Geometry: final body of the model. Coordinates: model frame, mm. A direction names the side the tool comes from. Give positions to 0.01 mm unless a question says otherwise; leave off trailing zeros. Write each loop counter-clockwise with the first axis right and the second up, starting at its lowest first coordinate (ties: lowest second). Pieces come first, ordered by that corner, then holes. Notation, with made-up numbers: M 19.25,-6 L 28.25,-6 A15 ccw 28.25,7 Z; hole C 14.5,55.25 d3. An arc over 180 degrees is marked long. Use one line per item in the form item = value. Start each with the question number.
Item 1: Section query C-C on z = -17. Return loops of the section in (x, y).
Item 2: Section query D-D on z = 0. Return loops of the section in (x, y).
Item 3: Section query A-A on x = -7. Return loops of the section in (y, z), then the cut area to 3 significant figures.
Item 4: Section query B-B on y = 4.25. Return loops of the section in (x, z).
Item 5: Access query for faces 4 (the flat face through (5, 0, 0)), 5 (the cylindrical face through (-4, -2, 0)), 6 (the flat face through (5, -0.5, -17.5)). Directions: +Z, -Z, +X, -X, +Y, -Y. A direction counts if a zero-diameter tool reaches every point of the face in a straight line with its end or side. Return the directions, or none.
Item 6: Pull-direction query (Y, two-part tool) for faces 1 (the flat face through (7, 0.1, 19)), 2 (the flat face through (-2, 0, 0)), 3 (the flat face through (0, 1, -5)); classes: released by +Y, released by -Y, zero draft, split by the parting line, or undercut.
Item 7: Contact query for flat-ended pins moving along their axis: P1, Ø1.5, axis at x = 3, z = 10.5, coming from the -Y side; P2, Ø4, axis at x = 8, z = -17.5, coming from the -Y side; P3, Ø1, axis at y = 4.5, z = -3.5, coming from the +X side. Output: stop coordinate, or through.
Item 8: Material intervals for line 1 along Z through (x, y) = (-2.75, 3); line 2 along X through (y, z) = (1.8, -17); line 3 along Z through (x, y) = (-3, 0), sorted ascending. Write a range as from..to.
from build123d import *

# Parameters (mm, degrees)
SKETCH_1_R          = 2
EXTRUDE_1_DEPTH     = 5
SKETCH_3_W          = 40
SKETCH_3_H          = 1.796813629
EXTRUDE_2_DEPTH     = 10
SKETCH_4_R          = 1.4
CUT_EXTRUDE_2_DEPTH = 20
SKETCH_6_R          = 2.5
EXTRUDE_3_DEPTH     = 7
SKETCH_7_R          = 2.8
SKETCH_7_R_2        = 2.2
CUT_EXTRUDE_3_DEPTH = 5
FILLET_1_R          = 1
EXTRUDE_START       = 5
SKETCH_8_W          = 5
SKETCH_8_H          = 4.9
SKETCH_8_R          = 1.4
EXTRUDE_4_DEPTH     = 5


with BuildPart() as part:
    # 스케치1 → 보스-돌출1 (new, symmetric)
    with BuildSketch(Plane(origin=(0, 0, 0), x_dir=(0, 0, -1), z_dir=(1, 0, 0))):
        Polygon((20, 6.896813629), (-20, 6.896813629), (-20, -1.103186371), (-15.1, -1.103186371), (-15.1, 5.1), (-5, 5.1), (-5, -3), (5, -3), (5, 5.1), (15.1, 5.1), (15.1, -1.103186371), (20, -1.103186371), align=None)
        Circle(SKETCH_1_R, mode=Mode.SUBTRACT)
    extrude(amount=EXTRUDE_1_DEPTH, both=True)

    # 스케치3 → 보스-돌출2 (add, symmetric)
    with BuildSketch(Plane(origin=(0, 0, 0), x_dir=(0, 0, -1), z_dir=(1, 0, 0))):
        with Locations((0, 5.998406815)):
            Rectangle(SKETCH_3_W, SKETCH_3_H)
    extrude(amount=EXTRUDE_2_DEPTH, both=True)

    # 스케치4 → 컷-돌출2 (cut)
    with BuildSketch(Plane(origin=(0, 0, 0), x_dir=(1, 0, 0), z_dir=(0, 1, 0))):
        with Locations(Location((-7, -17, 0), (0, 0, 90))):
            Circle(SKETCH_4_R)
        with Locations(Location((7, -17, 0), (0, 0, 90))):
            Circle(SKETCH_4_R)
        with Locations(Location((7, 17, 0), (0, 0, 90))):
            Circle(SKETCH_4_R)
        with Locations(Location((-7, 17, 0), (0, 0, 90))):
            Circle(SKETCH_4_R)
    extrude(amount=CUT_EXTRUDE_2_DEPTH, mode=Mode.SUBTRACT)

    # 스케치6 → 보스-돌출3 (add)
    with BuildSketch(Plane(origin=(5, 0, 0), x_dir=(0, 0, -1), z_dir=(1, 0, 0))):
        Circle(SKETCH_6_R)
    extrude(amount=-EXTRUDE_3_DEPTH)

    # 스케치7 → 컷-돌출3 (cut)
    with BuildSketch(Plane(origin=(5, 0, 0), x_dir=(0, 0, -1), z_dir=(1, 0, 0))):
        Circle(SKETCH_7_R)
        Circle(SKETCH_7_R_2, mode=Mode.SUBTRACT)
    extrude(amount=-CUT_EXTRUDE_3_DEPTH, mode=Mode.SUBTRACT)

    # 필렛1
    fillet_1_edges = [part.edges().sort_by_distance(p)[0] for p in [
        (5, 0, 2.2),
    ]]
    fillet(fillet_1_edges, radius=FILLET_1_R)

    # 스케치8 → 보스-돌출4 (add)
    # profile 1 of 4: a face of its own
    with BuildSketch(Plane.XZ.offset(-5.1).offset(EXTRUDE_START)):
        with Locations((-7.5, 17.55)):
            Rectangle(SKETCH_8_W, SKETCH_8_H)
        with Locations(Location((-7, 17, 0), (0, 0, 270))):
            Circle(SKETCH_8_R, mode=Mode.SUBTRACT)
    # profile 2 of 4: a face of its own
    with BuildSketch(Plane.XZ.offset(-5.1).offset(EXTRUDE_START)):
        with Locations((7.5, 17.55)):
            Rectangle(SKETCH_8_W, SKETCH_8_H)
        with Locations(Location((7, 17, 0), (0, 0, 270))):
            Circle(SKETCH_8_R, mode=Mode.SUBTRACT)
    # profile 3 of 4: a face of its own
    with BuildSketch(Plane.XZ.offset(-5.1).offset(EXTRUDE_START)):
        with Locations((-7.5, -17.55)):
            Rectangle(SKETCH_8_W, SKETCH_8_H)
        with Locations(Location((-7, -17, 0), (0, 0, 270))):
            Circle(SKETCH_8_R, mode=Mode.SUBTRACT)
    # profile 4 of 4: a face of its own
    with BuildSketch(Plane.XZ.offset(-5.1).offset(EXTRUDE_START)):
        with Locations((7.5, -17.55)):
            Rectangle(SKETCH_8_W, SKETCH_8_H)
        with Locations(Location((7, -17, 0), (0, 0, 270))):
            Circle(SKETCH_8_R, mode=Mode.SUBTRACT)
    extrude(amount=-EXTRUDE_4_DEPTH)


solid = part.part
Answer sheet:
q1.outline = M -10,0.1 L -8.4,0.1 L -8.4,6.9 L -10,6.9 Z; M -5.6,0.1 L -5,0.1 L -5,-1.1 L 5,-1.1 L 5,0.1 L 5.6,0.1 L 5.6,6.9 L -5.6,6.9 Z; M 8.4,0.1 L 10,0.1 L 10,6.9 L 8.4,6.9 Z
q2.outline = M -10,5.1 L -5,5.1 L -5,2 L -2,2 L -2,-2 L -5,-2 L -5,-3 L 5,-3 L 5,-2.8 L 0,-2.8 L 0,-2.2 L 4,-2.2 A1 ccw 5,-1.2 L 5,1.2 A1 ccw 4,2.2 L 0,2.2 L 0,2.8 L 5,2.8 L 5,5.1 L 10,5.1 L 10,6.9 L -10,6.9 Z
q3.outline = M 0.1,-20 L 6.9,-20 L 6.9,-18.4 L 0.1,-18.4 Z; M 0.1,-15.6 L 6.9,-15.6 L 6.9,15.6 L 0.1,15.6 L 0.1,15.1 L 5.1,15.1 L 5.1,-15.1 L 0.1,-15.1 Z; M 0.1,18.4 L 6.9,18.4 L 6.9,20 L 0.1,20 Z
q3.area = 82.8 mm2
q4.outline = M -10,-20 L 10,-20 L 10,-15.1 L -10,-15.1 Z; M -10,15.1 L 10,15.1 L 10,20 L -10,20 Z; M -5,-5 L 5,-5 L 5,5 L -5,5 Z; hole C -7,-17 d2.8; hole C -7,17 d2.8; hole C 7,-17 d2.8; hole C 7,17 d2.8
q5.face_4 = +X, -Y
q5.face_5 = -X
q5.face_6 = +Z, -Z, +X, -Y
q6.face_1 = released by -Y
q6.face_2 = undercut
q6.face_3 = zero draft
q7.P1 = 5.1
q7.P2 = 0.1
q7.P3 = 5
q8.line_1 = -20..-15.1, -5..5, 15.1..20
q8.line_2 = -10..-8.4, -5.6..5.6, 8.4..10
q8.line_3 = -20..-15.1, -5..-2, 2..5, 15.1..20
